Input: part model. Units: mm. Frame: model coordinates. A direction names the side the tool comes from. Round coordinates to 2 decimals unless told otherwise and drop trailing zeros. Loops run counter-clockwise (first coordinate to the right, second up) from the corner with the lowest first, then second, coordinate; pieces in that order, holes last. Notation, with made-up numbers: (-22, 69.25) -> (5, 69.25) arc R20 cw to (5, 102.25) -> close; hole circle Ø5 at (-4.5, 32.25). An arc over 180 degrees is marked (long way). Answer as a JSON object with one key per item and string values. Group by question number.
Item 1: Section query A-A on x = 0. Return loops of the section in (y, z), and give its area (3 significant figures).
Item 2: Pin query (flat end, axial travel): pin 1 (4.5 mm diameter, centred on x = 0, y = 22.02, fed in from -Z); pin 2 (1.5 mm diameter, centred on y = -7.5, z = 7, fed in from -X); pin 3 (4 mm diameter, centred on y = 22.5, z = 13, fed in from +X). Return the tip coordinate at first contact, or that it passes through.
Item 3: Section query D-D on x = -8. Return loops of the section in (y, z), and give its area (3 significant figures).
Item 4: Section query B-B on y = 0. Return loops of the section in (x, z), and give its area (3 significant figures).
Item 5: Material intervals for line 1 (Y direction, x = 0, z = 4.25); line 2 (Y direction, x = 0, z = 13.65); line 3 (Z direction, x = -19, y = -12), sorted ascending. Write a range as [from, to].
Item 6: Set-up query: faces 4 (the cylindrical face through (-7.34, -33.04, 5.36)), 5 (the flat face through (20, -31, 0.711)), 6 (the cylindrical face through (-0.88, -20.34, 13.49)). Return all of +Z, -Z, +X, -X, +Y, -Y with unobstructed straight access to the full face (end or side cutting, diameter ignored); none if empty.
Item 7: Draft query along X for faces 1 (the cylindrical face through (-28.915, -22.171, 8.262)), 2 (the flat face through (-26, -22, 0)), 3 (the cylindrical face through (0.25, 20.14, 13.49)). Return one class per face: released by +X, released by -X, zero draft, split by the parting line, or undercut.
Item 8: Section query C-C on z = 6.5. Return loops of the section in (x, y).
from build123d import *

# Parameters (mm, degrees)
F0_R     = 38.0619
F0_R_2   = 36.4363
F1_DEPTH = 0.7112
F0_R_3   = 33.8455
F2_DEPTH = 16.0274
F3_DEPTH = 10.8712
F5_D     = 3.7973


with BuildPart() as f1:
    # F0 (on Top) → F1 (new body)
    with BuildSketch(Plane.XY):
        Circle(F0_R)
        Circle(F0_R_2, mode=Mode.SUBTRACT)
    extrude(amount=F1_DEPTH)

    # F0 (on Top) → F2 (join)
    with BuildSketch(Plane.XY):
        Circle(F0_R_2)
        Circle(F0_R_3, mode=Mode.SUBTRACT)
        Circle(F0_R_3)
    extrude(amount=F2_DEPTH)

    # F0 (on Top) → F3 (cut)
    with BuildSketch(Plane.XY):
        Circle(F0_R_3)
    extrude(amount=F3_DEPTH, mode=Mode.SUBTRACT)

    # F5 (through all)
    with Locations(Plane(origin=(0, 0, 0), x_dir=(1, 0, 0), z_dir=(0, 0, -1))):
        with Locations((0, 22.0218), (0, -22.0218)):
            Hole(F5_D / 2)


solid = f1.part
Solved:
{
 "1": {"outline": "(-38.06, 0) -> (-33.85, 0) -> (-33.85, 10.87) -> (-23.92, 10.87) -> (-23.92, 16.03) -> (-36.44, 16.03) -> (-36.44, 0.71) -> (-38.06, 0.71) -> close; (-20.12, 10.87) -> (20.12, 10.87) -> (20.12, 16.03) -> (-20.12, 16.03) -> close; (23.92, 10.87) -> (33.85, 10.87) -> (33.85, 0) -> (38.06, 0) -> (38.06, 0.71) -> (36.44, 0.71) -> (36.44, 16.03) -> (23.92, 16.03) -> close", "area": "395 mm²"},
 "2": {"pin 1": "z = 10.87", "pin 2": "x = -35.81", "pin 3": "x = 30.12"},
 "3": {"outline": "(-37.21, 0) -> (-32.89, 0) -> (-32.89, 10.87) -> (32.89, 10.87) -> (32.89, 0) -> (37.21, 0) -> (37.21, 0.71) -> (35.55, 0.71) -> (35.55, 16.03) -> (-35.55, 16.03) -> (-35.55, 0.71) -> (-37.21, 0.71) -> close", "area": "427 mm²"},
 "4": {"outline": "(-38.06, 0) -> (-33.85, 0) -> (-33.85, 10.87) -> (33.85, 10.87) -> (33.85, 0) -> (38.06, 0) -> (38.06, 0.71) -> (36.44, 0.71) -> (36.44, 16.03) -> (-36.44, 16.03) -> (-36.44, 0.71) -> (-38.06, 0.71) -> close", "area": "434 mm²"},
 "5": {"line 1": "[-36.44, -33.85], [33.85, 36.44]", "line 2": "[-36.44, -23.92], [-20.12, 20.12], [23.92, 36.44]", "line 3": "[10.87, 16.03]"},
 "6": {"face 4": "-Z", "face 5": "+Z", "face 6": "+Z, -Z"},
 "7": {"face 1": "split by the parting line", "face 2": "zero draft", "face 3": "undercut"},
 "8": {"outline": "circle Ø72.87 at (0, 0); hole circle Ø67.69 at (0, 0)"}
}
